Input: part model. Units: mm. Frame: model coordinates. Face numbers are marked on the shaded views. Coordinates: 2 decimals unless noted, no trailing zeros. Loops run counter-clockwise (first coordinate to the right, second up) from the corner with the lowest first, then second, coordinate; pieces in that order, holes last.
Item 1: Section C-C on x = -31. Return loops of the section in (y, z).
Item 2: Section A-A on y = 0. Give the number of separate pieces and of enclosed holes in the cut face, and give its area (3 significant figures).
Item 3: Contact query for flat-ended pins moving along their axis: P1, Ø10, axis at x = -22.5, z = 5, coming from the -Y side; P2, Ø6, axis at y = 19, z = 16.5, coming from the -X side. Output: stop coordinate, or through.
Item 4: Ray query, line 1 along X through (y, z) = (-15.5, 12.5); line 2 along Y through (x, z) = (-13.5, 5.5); line 3 along Y through (x, z) = (45, 11.5). Return the intervals inside material, ascending.
Item 5: Pull-direction query (X, two-part tool) for the marked faces 1 and 2; classes: released by +X, released by -X, zero draft, split by the parting line, or undercut.
```python
from build123d import *

# Parameters (mm, degrees)
F0_R     = 6.9174599135
F0_R_2   = 6.6953536728
F1_DEPTH = 33.02


with BuildPart() as f1:
    # F0 (on Top) → F1 (new body)
    with BuildSketch(Plane.XY):
        with BuildLine():
            ThreePointArc((13.6920073452, -41.4780412298), (23.9509627201, -44.6805622966), (29.0285234771, -35.2084620371))
            add(Edge.make_bspline(
                [(29.0285234771, -35.2084620371), (68.2918037486, -11.4532756006), (42.3845917945, 23.2317086668)],
                knots=[5.3273150829, 5.3273150829, 5.3273150829, 6.8523899746, 6.8523899746, 6.8523899746], degree=2, weights=[1, 0.7230855783, 1]))
            ThreePointArc((42.3845917945, 23.2317086668), (44.3217640549, 45.8550598259), (22.8771801048, 38.3919188491))
            add(Edge.make_bspline(
                [(22.8771801048, 38.3919188491), (-2.5443945173, 49.5081889699), (-26.727217642, 36.5211438216)],
                knots=[1.0988176954, 1.0988176954, 1.0988176954, 2.1307691564, 2.1307691564, 2.1307691564], degree=2, weights=[1, 0.8698117268, 1]))
            ThreePointArc((-26.727217642, 36.5211438216), (-48.2228883846, 41.3370667245), (-44.8327850103, 19.5709422832))
            add(Edge.make_bspline(
                [(-44.8327850103, 19.5709422832), (-62.9066905476, -10.8120093087), (-32.5500646686, -32.8710234635)],
                knots=[2.6703042477, 2.6703042477, 2.6703042477, 4.0088984161, 4.0088984161, 4.0088984161], degree=2, weights=[1, 0.7842579731, 1]))
            ThreePointArc((-32.5500646686, -32.8710234635), (-26.1357518543, -43.7893377337), (-13.6851041212, -41.479713))
            add(Edge.make_bspline(
                [(-13.6851041212, -41.479713), (0.0037274647, -44.7938672304), (13.6920073452, -41.4780412298)],
                knots=[4.4369485173, 4.4369485173, 4.4369485173, 4.9879720114, 4.9879720114, 4.9879720114], degree=2, weights=[1, 0.9622861083, 1]))
        make_face()
        with Locations((-19.0128814429, 0)):
            Circle(F0_R, mode=Mode.SUBTRACT)
        with BuildLine():
            add(Edge.make_bspline(
                [(-4.6130437404, -10.112545453), (-2.8805919387, -7.2566060297), (10.8589562819, -6.9282740006), (-0.1500027257, -23.178328073), (-6.2456456393, -12.8038827364), (-4.6130437404, -10.112545453)],
                knots=[0, 0, 0, 0, 0.3419572904, 0.6777514266, 1, 1, 1, 1], degree=3))
        make_face(mode=Mode.SUBTRACT)
        with Locations((14.8867378011, 0)):
            Circle(F0_R_2, mode=Mode.SUBTRACT)
    extrude(amount=F1_DEPTH)


solid = f1.part
```
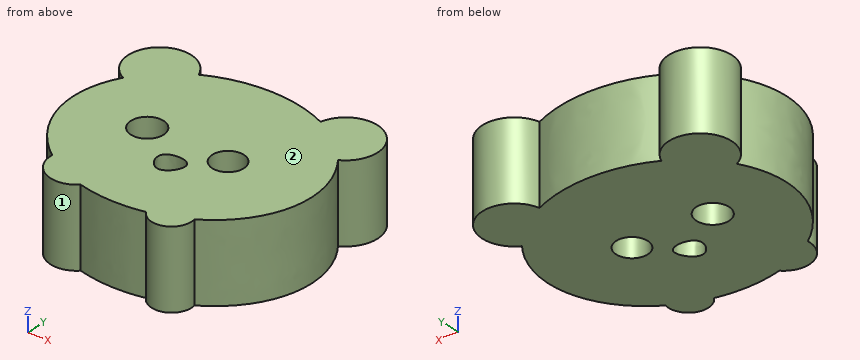
Results found:
1. outline: (-39.45, 0) - (42.18, 0) - (42.18, 33.02) - (-39.45, 33.02) - close
2. separate pieces: 3
2. enclosed holes: 0
2. area: 2,420 mm2
3. P1: stops at y = -44.78
3. P2: stops at x = -48.35
4. line 1: x = -46.95 to -3.83, 4.16 to 46.95
4. line 2: y = -41.52 to -4.18, 4.18 to 41.52
4. line 3: y = -19.29 to 19.29, 25.05 to 45.29
5. face 1: undercut
5. face 2: zero draft
